```python
from build123d import *

# Parameters (mm, degrees)
CYLINDER032_R     = 2
CYLINDER032_DEPTH = 10
CYLINDER030_R     = 3
CYLINDER030_DEPTH = 10
CYLINDER031_R     = 5
CYLINDER031_DEPTH = 6
FILLET008_R       = 1


with BuildPart() as hole_cylinder:
    # Cylinder032 → Cylinder032 (new body)
    with BuildSketch(Plane.XY):
        Circle(CYLINDER032_R)
    extrude(amount=CYLINDER032_DEPTH)


with BuildPart() as fusion010:
    # Cylinder030 → Cylinder030 (new body)
    with BuildSketch(Plane.XY.offset(1)):
        Circle(CYLINDER030_R)
    extrude(amount=CYLINDER030_DEPTH)

    # Fusion010: union hole cylinder
    add(hole_cylinder.part)


with BuildPart() as fillet008:
    # Cylinder031 → Cylinder031 (new body)
    with BuildSketch(Plane.XY):
        Circle(CYLINDER031_R)
    extrude(amount=CYLINDER031_DEPTH)

    # Cut012: cut Fusion010
    add(fusion010.part, mode=Mode.SUBTRACT)

    # Fillet008
    fillet008_edges = [fillet008.edges().sort_by_distance(p)[0] for p in [
        (-5, 0, 6),
    ]]
    fillet(fillet008_edges, radius=FILLET008_R)


solid = fillet008.part
```
Can you work these out from the model? Positions are in its coordinate system, mm. A direction names the side the tool comes from. Coordinates: 2 decimals unless noted, no trailing zeros. Order: outer loops, then holes, each group sorted by start corner. A loop starts at its lowest first (then second) coordinate and runs counter-clockwise, first axis right, second up. Notation, with made-up numbers: (65, -15) - (83, -15) arc R12 ccw to (83, 4) - close; hole circle Ø4 at (18.25, 66.25). An arc over 180 degrees is marked (long way). Answer in a Markdown table with one row per item.
1. Suppose I cut it at C-C (z = 2.3). Please give me the cut outline in (x, y), and give its area (3 significant figures).
Reply:
| item | result |
|---|---|
| outline | circle Ø10 at (0, 0); hole circle Ø6 at (0, 0) |
| area | 50.3 mm^2 |
2. For pin 1 (1 mm diameter, centred on x = 4, y = 3, fed in from +Z); pin 2 (3 mm diameter, centred on x = 0, y = 0, fed in from +Z); pin 3 (1 mm diameter, centred on x = -3.5, z = 4.5, fed in from -Y); pin 4 (1.5 mm diameter, centred on y = 1, z = 1.5, fed in from -X), each with a flat end and sliding along its axis, tell me the tip position at first contact or that it passes through.
Reply:
| item | result |
|---|---|
| pin 1 | stops at z = 5.87 |
| pin 2 | passes through |
| pin 3 | stops at y = -4 |
| pin 4 | stops at x = -4.99 |
3. If I drill on line 1 along Y through (x, z) = (0, 0.65); line 2 along Y through (x, z) = (0, 4.3); line 3 along Z through (x, y) = (-1.75, -1.25), over which ranges is the centre line in solid material (lowest first)?
Reply:
| item | result |
|---|---|
| line 1 | y = -5 to -2, 2 to 5 |
| line 2 | y = -5 to -3, 3 to 5 |
| line 3 | z = 0 to 1 |
4. For faces 1 (the flat face through (1, -2, 1)), 2 (the flat face through (-0.1, -2.2, 0)), which set-ups out of +Z, -Z, +X, -X, +Y, -Y let a thin tool reach every point of the face, with its end or its side?
Reply:
| item | result |
|---|---|
| face 1 | +Z |
| face 2 | -Z, +X, -X, +Y, -Y |
5. Suppose I cut it at A-A (x = 0). Please give me the cut outline in (y, z), and give its area (3 significant figures).
Reply:
| item | result |
|---|---|
| outline | (-5, 0) - (-2, 0) - (-2, 1) - (-3, 1) - (-3, 6) - (-4, 6) arc R1 ccw to (-5, 5) - close; (2, 0) - (5, 0) - (5, 5) arc R1 ccw to (4, 6) - (3, 6) - (3, 1) - (2, 1) - close |
| area | 25.6 mm^2 |
6. If we mould it in two halves opening along X, with no side actions, what happens to faces 3 (the cylindrical face through (-1.08, -4.88, 2.46)), 4 (the cylindrical face through (-0.434, -1.952, 0.493)), 5 (the flat face through (1, 3, 6)), 6 (the cylindrical face through (-3, 0, 3))? For each: pulls with the +X half, pulls with the -X half, needs draft (parallel to the pull), parting line crosses it, or undercut.
Reply:
| item | result |
|---|---|
| face 3 | parting line crosses it |
| face 4 | undercut |
| face 5 | needs draft |
| face 6 | undercut |
7. Suppose I cut it at D-D (z = 5.4). Please give me the cut outline in (x, y), and give its area (3 significant figures).
Reply:
| item | result |
|---|---|
| outline | circle Ø9.83 at (0, 0); hole circle Ø6 at (0, 0) |
| area | 47.7 mm^2 |
